from build123d import *

# Parameters (mm, degrees)
SKETCH1_W           = 40
SKETCH1_H           = 40
BOSS_EXTRUDE1_DEPTH = 5
SKETCH2_R           = 4
SKETCH2_R_2         = 1.5
BOSS_EXTRUDE2_DEPTH = 40
SKETCH4_R           = 1.5
CUT_EXTRUDE1_DEPTH  = 40
SKETCH5_W           = 9.64553252
SKETCH5_H           = 8.977750056
CUT_EXTRUDE3_DEPTH  = 10
SKETCH6_W           = 13.188128002
SKETCH6_H           = 14.056051126
CUT_EXTRUDE4_DEPTH  = 10
SKETCH8_R           = 1
CUT_EXTRUDE5_DEPTH  = 7.5
SKETCH9_W           = 20.740982478
SKETCH9_H           = 15
CUT_EXTRUDE6_DEPTH  = 7.5
SKETCH16_R          = 4.5
BOSS_EXTRUDE3_DEPTH = 20
SKETCH17_R          = 2
CUT_EXTRUDE7_DEPTH  = 20


with BuildPart() as part:
    # Sketch1 → Boss-Extrude1 (new body)
    with BuildSketch(Plane(origin=(0, 0, 0), x_dir=(0, 0, -1), z_dir=(1, 0, 0))):
        Rectangle(SKETCH1_W, SKETCH1_H)
    extrude(amount=BOSS_EXTRUDE1_DEPTH)

    # Sketch2 → Boss-Extrude2 (add)
    with BuildSketch(Plane.XY.offset(20)):
        with Locations((2.5, -20)):
            Circle(SKETCH2_R)
        with Locations((2.5, -20)):
            Circle(SKETCH2_R_2, mode=Mode.SUBTRACT)
    extrude(amount=-BOSS_EXTRUDE2_DEPTH)

    # Sketch4 → Cut-Extrude1 (cut)
    with BuildSketch(Plane.XY.offset(20)):
        with Locations((2.5, -20)):
            Circle(SKETCH4_R)
    extrude(amount=-CUT_EXTRUDE1_DEPTH, mode=Mode.SUBTRACT)

    # Sketch5 → Cut-Extrude3 (cut)
    with BuildSketch(Plane(origin=(0, 0, -20), x_dir=(-1, 0, 0), z_dir=(0, 0, -1))):
        with Locations((-2.5, -21.5)):
            Rectangle(SKETCH5_W, SKETCH5_H)
    extrude(amount=-CUT_EXTRUDE3_DEPTH, mode=Mode.SUBTRACT)

    # Sketch6 → Cut-Extrude4 (cut)
    with BuildSketch(Plane.XY.offset(20)):
        with Locations((2.5, -24)):
            Rectangle(SKETCH6_W, SKETCH6_H)
    extrude(amount=-CUT_EXTRUDE4_DEPTH, mode=Mode.SUBTRACT)

    # Sketch8 → Cut-Extrude5 (cut, through all)
    with BuildSketch(Plane(origin=(5, 0, 0), x_dir=(0, 0, -1), z_dir=(1, 0, 0))):
        with Locations((-10.5, 16.5612495)):
            Circle(SKETCH8_R)
        with Locations((10.5, 16.5612495)):
            Circle(SKETCH8_R)
        with Locations((10.5, 3.5612495)):
            Circle(SKETCH8_R)
        with Locations((-10.5, 3.5612495)):
            Circle(SKETCH8_R)
    extrude(amount=-CUT_EXTRUDE5_DEPTH, mode=Mode.SUBTRACT)

    # Sketch9 → Cut-Extrude6 (cut, through all)
    with BuildSketch(Plane(origin=(5, 0, 0), x_dir=(0, 0, -1), z_dir=(1, 0, 0))):
        with Locations((0, -6.471626191)):
            Rectangle(SKETCH9_W, SKETCH9_H)
    extrude(amount=-CUT_EXTRUDE6_DEPTH, mode=Mode.SUBTRACT)

    # Sketch16 → Boss-Extrude3 (add)
    with BuildSketch(Plane.XY.offset(10)):
        with Locations((2.5, -20)):
            Circle(SKETCH16_R)
    extrude(amount=-BOSS_EXTRUDE3_DEPTH)

    # Sketch17 → Cut-Extrude7 (cut)
    with BuildSketch(Plane.XY.offset(10)):
        with Locations((2.5, -20)):
            Circle(SKETCH17_R)
    extrude(amount=-CUT_EXTRUDE7_DEPTH, mode=Mode.SUBTRACT)


solid = part.part
The listing builds one solid part. Answer for the finished solid, in the listing's coordinates (mm). A direction names the side the tool comes from. Round coordinates to 2 decimals unless told otherwise and drop trailing zeros. Order: outer loops, then holes, each group sorted by start corner. A loop starts at its lowest first (then second) coordinate and runs counter-clockwise, first axis right, second up. Notation, with made-up numbers: M 71,82 L 90,82 A21 cw 90,119 Z; hole C 19,34 d7. An arc over 180 degrees is marked long. Answer in a Markdown table with one row per item. Add a question column.
1) The part is cut by section A-A on z = 5. Determine the outline of the cut face in (x, y).
2) Determine the mould class of faces 1 (the face through (2.535, 15.585, 10.717)), 2 (the face through (2.4, -22.2, 10)), 3 (the face through (2, 20, 0)) for opening direction Z: pulls with the +Z half, pulls with the -Z half, needs draft (parallel to the pull), parting line crosses it, or undercut.
3) Consider line 1 along Y through (x, z) = (1.05, -10.5); line 2 along Y through (x, z) = (2.5, 6); line 3 along X through (y, z) = (-14, -13.5). Determine where each line is inside the solid, lowest interval first. Write a range as from..to.
4) The part is cut by section C-C on x = 2.5. Determine the outline of the cut face in (y, z), plus the area to 3 significant figures.
5) Which of the six approach directions +Z, -Z, +X, -X, +Y, -Y give full straight-line access (tool end or side, diameter ignored) to faces 4 (the face through (3, -17.011, -15)), 5 (the face through (2.24, -18.017, 0.14)), 6 (the face through (2, -16.972, 15)), 7 (the face through (3, 1.028, 0)), 8 (the face through (2, 2, -20))?
6) The part is cut by section B-B on y = -12.5. Determine the outline of the cut face in (x, z), plus the area to 3 significant figures.
7) The part is cut by section D-D on z = 13. Determine the outline of the cut face in (x, y), plus the area to 3 significant figures.
8) Flat-ended cylindrical pins translate along their axes: pin 1 Ø1.5 at (x, z) = (2, -16) entering from -Y; pin 2 Ø3.5 at (x, y) = (2.5, -20) entering from +Z; pin 3 Ø18.5 at (y, z) = (-2, -2) entering from +X; pin 4 Ø2.5 at (x, y) = (3, -18.5) entering from +Z. Find the tip coordinate at first contact, or state that the pin passes through.
Findings below:
| question | item | result |
|---|---|---|
| 1 | outline | M 0,-16.26 A4.5 ccw long 5,-16.26 L 5,-13.97 L 0,-13.97 Z; M 0,1.03 L 5,1.03 L 5,20 L 0,20 Z; hole C 2.5,-20 d4 |
| 2 | face 1 | undercut |
| 2 | face 2 | pulls with the +Z half |
| 2 | face 3 | needs draft |
| 3 | line 1 | y = -17.01..2.56, 4.56..15.56, 17.56..20 |
| 3 | line 2 | y = -24.5..-22, -18..-13.97, 1.03..20 |
| 3 | line 3 | x = 0..5 |
| 4 | outline | M -24.5,-10 L -22,-10 L -22,10 L -24.5,10 Z; M -18,-10 L -17.01,-10 L -17.01,-20 L 20,-20 L 20,20 L -16.97,20 L -16.97,10 L -18,10 Z; hole M -13.97,-10.37 L 1.03,-10.37 L 1.03,10.37 L -13.97,10.37 Z; hole C 3.56,-10.5 d2; hole C 3.56,10.5 d2; hole C 16.56,-10.5 d2; hole C 16.56,10.5 d2 |
| 4 | area | 1,230 mm² |
| 5 | face 4 | -Z, +X, -X, -Y |
| 5 | face 5 | +Z, -Z |
| 5 | face 6 | +Z, +X, -X, -Y |
| 5 | face 7 | +X, -X |
| 5 | face 8 | -Z, +X, -X, +Y, -Y |
| 6 | outline | M 0,-20 L 5,-20 L 5,-10.37 L 0,-10.37 Z; M 0,10.37 L 5,10.37 L 5,20 L 0,20 Z |
| 6 | area | 96.3 mm² |
| 7 | outline | M -0.11,-16.97 L 5.11,-16.97 A4 ccw 5,-16.88 L 5,20 L 0,20 L 0,-16.88 A4 ccw Z |
| 7 | area | 185 mm² |
| 8 | pin 1 | stops at y = -17.01 |
| 8 | pin 2 | passes through |
| 8 | pin 3 | stops at x = 5 |
| 8 | pin 4 | stops at z = 10 |
